Verification items for the finished model (mm, model axes). A direction names the side the tool comes from. Give positions to 0.01 mm unless a question says otherwise; leave off trailing zeros. Write each loop counter-clockwise with the first axis right and the second up, starting at its lowest first coordinate (ties: lowest second). Pieces come first, ordered by that corner, then holes. Notation, with made-up numbers: M 40.25,20 L 90.25,20 A10 ccw 90.25,25 Z; hole C -3.5,-1.75 d8. An arc over 180 degrees is marked long. Answer as a JSON object with one key per item and string values.
```python
from build123d import *

# Parameters (mm, degrees)
EXTRUSION1_DEPTH = 5.9


with BuildPart() as part:
    # Esquisse1 → Extrusion1 (new body)
    with BuildSketch(Plane.XY):
        with BuildLine():
            Line((0, 0), (15, 0))
            Line((15, 0), (15, 7.4))
            ThreePointArc((15, 7.4), (7.5, 14.9), (0, 7.4))
            Line((0, 7.4), (0, 0))
        make_face()
        with BuildLine():
            Line((6.173350084, 8.91), (8.826649916, 8.91))
            ThreePointArc((8.826649916, 8.91), (9.51, 7.4), (8.826649916, 5.89))
            Line((8.826649916, 5.89), (6.173350084, 5.89))
            ThreePointArc((6.173350084, 5.89), (5.49, 7.4), (6.173350084, 8.91))
        make_face(mode=Mode.SUBTRACT)
    extrude(amount=EXTRUSION1_DEPTH)


solid = part.part
```
1) Release check for a two-part mould opening along Y. For faces 3 (the face through (5.49, 7.38, 2.91)), 4 (the face through (7, 0, 3)), 5 (the face through (0, 4, 3)) record: pulls with the +Y half, pulls with the -Y half, needs draft (parallel to the pull), parting line crosses it, or undercut.
Completed:
{"face 3": "undercut", "face 4": "pulls with the -Y half", "face 5": "needs draft"}
2) Section check D-D on x = 10.75. Record the boundary of the cut face in (y, z).
Completed:
{"outline": "M 0,0 L 14.16,0 L 14.16,5.9 L 0,5.9 Z"}
3) Go/stop test with flat-tipped pins: pin 1 (1.5 mm diameter, centred on x = 10, z = 1.5, fed in from +Y); pin 2 (4 mm diameter, centred on x = 7, y = 6.5, fed in from -Z). Record where each tip stops, or that it passes through.
Completed:
{"pin 1": "stops at y = 14.69", "pin 2": "stops at z = 0"}
4) Section check A-A on x = 7.5. Record the boundary of the cut face in (y, z), and give its area (3 significant figures).
Completed:
{"outline": "M 0,0 L 5.89,0 L 5.89,5.9 L 0,5.9 Z; M 8.91,0 L 14.9,0 L 14.9,5.9 L 8.91,5.9 Z", "area": "70.1 mm2"}
5) Section check B-B on z = 3. Record the boundary of the cut face in (x, y), and give its area (3 significant figures).
Completed:
{"outline": "M 0,0 L 15,0 L 15,7.4 A7.5 ccw 0,7.4 Z; hole M 6.17,5.89 L 8.83,5.89 A2.01 ccw 8.83,8.91 L 6.17,8.91 A2.01 ccw Z", "area": "188 mm2"}
6) Section check C-C on y = 6.5. Record the boundary of the cut face in (x, z).
Completed:
{"outline": "M 0,0 L 5.7,0 L 5.7,5.9 L 0,5.9 Z; M 9.3,0 L 15,0 L 15,5.9 L 9.3,5.9 Z"}
7) Thickness scan on L1, parallel to Y at x = 7.25, z = 0.6; L2, parallel to Y at x = 6.25, z = 3.2; L3, parallel to X at y = 7.25, z = 3.75. Record the ranges inside material, lowest first.
Completed:
{"L1": "y = 0 to 5.89, 8.91 to 14.9", "L2": "y = 0 to 5.89, 8.91 to 14.8", "L3": "x = 0 to 5.5, 9.5 to 15"}
8) Access from +Z, -Z, +X, -X, +Y, -Y to the whole of each face (thin tool, end or side, straight path). Record for faces 1 (the face through (15, 4, 3)), 2 (the face through (8, 5.89, 3)).
Completed:
{"face 1": "+Z, -Z, +X, +Y, -Y", "face 2": "+Z, -Z"}
